from build123d import *

# Parameters (mm, degrees)
SKETCH_1_W          = 104
SKETCH_1_H          = 135
SKETCH_1_R          = 47
EXTRUDE_2_DEPTH     = 100
SKETCH_2_W          = 94
SKETCH_2_H          = 94
CUT_EXTRUDE_1_DEPTH = 95
SKETCH_3_W          = 30
SKETCH_3_H          = 5
SKETCH_3_W_2        = 94
SKETCH_3_H_2        = 20
CUT_EXTRUDE_3_DEPTH = 70
SKETCH_4_W          = 20
SKETCH_4_H          = 4
SKETCH_4_W_2        = 4
SKETCH_4_H_2        = 20
CUT_EXTRUDE_4_DEPTH = 10
CUT_EXTRUDE_6_REACH = 106
SKETCH_6_W          = 55
SKETCH_6_H          = 17
CUT_EXTRUDE_7_REACH = 137
SKETCH_7_W          = 12
SKETCH_7_H          = 12


with BuildPart() as part:
    # 草圖1 → 填料-伸長2 (new body)
    with BuildSketch(Plane.XY):
        with Locations((-20.894077044, -18.213740458)):
            Rectangle(SKETCH_1_W, SKETCH_1_H)
        with Locations((-20.894077044, -7.713740458)):
            Circle(SKETCH_1_R, mode=Mode.SUBTRACT)
    extrude(amount=EXTRUDE_2_DEPTH)

    # 草圖2 → 除料-伸長1 (cut)
    with BuildSketch(Plane.XY.offset(100)):
        with Locations((-20.894077044, -7.713740458)):
            Rectangle(SKETCH_2_W, SKETCH_2_H)
    extrude(amount=-CUT_EXTRUDE_1_DEPTH, mode=Mode.SUBTRACT)

    # 草圖3 → 除料-伸長3 (cut)
    with BuildSketch(Plane.XY.offset(100)):
        with Locations((11.105922956, -57.213740458)):
            Rectangle(SKETCH_3_W, SKETCH_3_H)
        with Locations((-20.894077044, -69.713740458)):
            Rectangle(SKETCH_3_W_2, SKETCH_3_H_2)
    extrude(amount=-CUT_EXTRUDE_3_DEPTH, mode=Mode.SUBTRACT)

    # 草圖4 → 除料-伸長4 (cut)
    with BuildSketch(Plane.XY.offset(100)):
        with Locations((-15.894077044, -81.713740458)):
            Rectangle(SKETCH_4_W, SKETCH_4_H)
        with Locations((28.105922956, -8.713740458)):
            Rectangle(SKETCH_4_W_2, SKETCH_4_H_2)
        with Locations((-15.894077044, 41.286259542)):
            Rectangle(SKETCH_4_W, SKETCH_4_H)
    extrude(amount=-CUT_EXTRUDE_4_DEPTH, mode=Mode.SUBTRACT)

    # 草圖6 → 除料-伸長6 (cut, up to next)
    with BuildSketch(Plane.ZY.offset(72.894077044), mode=Mode.PRIVATE) as cut_extrude_6_sk1:
        with Locations((62.5, 22.786259542)):
            Rectangle(SKETCH_6_W, SKETCH_6_H)
    cut_extrude_6_tool1 = extrude(cut_extrude_6_sk1.sketch, amount=-CUT_EXTRUDE_6_REACH, mode=Mode.PRIVATE) & part.part
    add(cut_extrude_6_tool1.solids().sort_by_distance((-72.894077, 22.78626, 62.5))[0], mode=Mode.SUBTRACT)
    # 草圖6 → 除料-伸長6 (cut, up to next)
    with BuildSketch(Plane.ZY.offset(72.894077044), mode=Mode.PRIVATE) as cut_extrude_6_sk2:
        with Locations((62.5, 1.786259542)):
            Rectangle(SKETCH_6_W, SKETCH_6_H)
    cut_extrude_6_tool2 = extrude(cut_extrude_6_sk2.sketch, amount=-CUT_EXTRUDE_6_REACH, mode=Mode.PRIVATE) & part.part
    add(cut_extrude_6_tool2.solids().sort_by_distance((-72.894077, 1.78626, 62.5))[0], mode=Mode.SUBTRACT)
    # 草圖6 → 除料-伸長6 (cut, up to next)
    with BuildSketch(Plane.ZY.offset(72.894077044), mode=Mode.PRIVATE) as cut_extrude_6_sk3:
        with Locations((62.5, -19.213740458)):
            Rectangle(SKETCH_6_W, SKETCH_6_H)
    cut_extrude_6_tool3 = extrude(cut_extrude_6_sk3.sketch, amount=-CUT_EXTRUDE_6_REACH, mode=Mode.PRIVATE) & part.part
    add(cut_extrude_6_tool3.solids().sort_by_distance((-72.894077, -19.21374, 62.5))[0], mode=Mode.SUBTRACT)
    # 草圖6 → 除料-伸長6 (cut, up to next)
    with BuildSketch(Plane.ZY.offset(72.894077044), mode=Mode.PRIVATE) as cut_extrude_6_sk4:
        with Locations((62.5, -40.213740458)):
            Rectangle(SKETCH_6_W, SKETCH_6_H)
    cut_extrude_6_tool4 = extrude(cut_extrude_6_sk4.sketch, amount=-CUT_EXTRUDE_6_REACH, mode=Mode.PRIVATE) & part.part
    add(cut_extrude_6_tool4.solids().sort_by_distance((-72.894077, -40.21374, 62.5))[0], mode=Mode.SUBTRACT)

    # 草圖7 → 除料-伸長7 (cut, up to next)
    with BuildSketch(Plane.XZ.offset(85.713740458), mode=Mode.PRIVATE) as cut_extrude_7_sk1:
        with Locations((5.105922956, 49)):
            Rectangle(SKETCH_7_W, SKETCH_7_H)
    cut_extrude_7_tool1 = extrude(cut_extrude_7_sk1.sketch, amount=-CUT_EXTRUDE_7_REACH, mode=Mode.PRIVATE) & part.part
    add(cut_extrude_7_tool1.solids().sort_by_distance((5.105923, -85.71374, 49))[0], mode=Mode.SUBTRACT)
    # 草圖7 → 除料-伸長7 (cut, up to next)
    with BuildSketch(Plane.XZ.offset(85.713740458), mode=Mode.PRIVATE) as cut_extrude_7_sk2:
        with Locations((-46.894077044, 49)):
            Rectangle(SKETCH_7_W, SKETCH_7_H)
    cut_extrude_7_tool2 = extrude(cut_extrude_7_sk2.sketch, amount=-CUT_EXTRUDE_7_REACH, mode=Mode.PRIVATE) & part.part
    add(cut_extrude_7_tool2.solids().sort_by_distance((-46.894077, -85.71374, 49))[0], mode=Mode.SUBTRACT)


solid = part.part
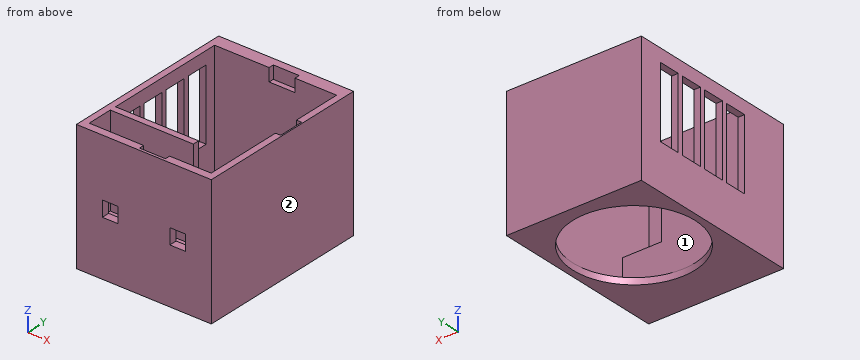
For this review, take the finished solid that the model builds, in its own axes (mm). Face numbers are marked on the shaded views. A direction names the side the tool comes from. Round coordinates to 2 decimals unless told otherwise and drop trailing zeros. Write each loop counter-clockwise with the first axis right and the second up, starting at its lowest first coordinate (ties: lowest second). Pieces come first, ordered by that corner, then holes. Notation, with made-up numbers: M 37.5,-39 L 50.5,-39 A21 cw 50.5,-21 Z; hole C 69.5,29.25 d2. An arc over 180 degrees is marked long. Write item = value, one per line. Start each with the question number.
(1) We need section C-C (x = -48). Give the boundary of the cut face in (y, z).
(2) For line 1 along Y through (x, z) = (-42, 66); line 2 along Y through (x, z) = (24, 22); line 3 along X through (y, z) = (-65, 71), list the stretches that pass through material, from the lowest coordinate up.
(3) We need section B-B (y = -34.5). Give the boundary of the cut face in (x, z), then the cut area to 3 significant figures.
(4) Clearance check with flat-ended pins moving along their axes: pin 1 Ø3 at (y, z) = (18.5, 44.5) entering from -X; pin 2 Ø3 at (x, y) = (-44.5, -81.5) entering from -Z. State where each tip first meets the part, or that it passes through.
(5) We need section D-D (z = 16). Give the boundary of the cut face in (x, y).
(6) For the marked faces 1 and 2, list the 3-axis set-ups (+Z, -Z, +X, -X, +Y, -Y) from which the entire face can be reached by the end or side of a thin tool; tool diameter is ignored.
(7) We need section A-A (z = 59.5). Give the boundary of the cut face in (x, y), then the cut area to 3 significant figures.
Results found:
q1.outline = M -85.71,0 L -46.11,0 L -46.11,5 L -54.71,5 L -54.71,100 L -59.71,100 L -59.71,30 L -79.71,30 L -79.71,43 L -85.71,43 Z; M -85.71,55 L -79.71,55 L -79.71,100 L -85.71,100 Z; M 30.68,0 L 49.29,0 L 49.29,100 L 39.29,100 L 39.29,5 L 30.68,5 Z
q2.line_1 = -85.71 to -79.71, -59.71 to -54.71, 39.29 to 49.29
q2.line_2 = -85.71 to -54.71, 39.29 to 49.29
q2.line_3 = -72.89 to -67.89, 26.11 to 31.11
q3.outline = M -72.89,0 L -59.51,0 L -59.51,5 L -67.89,5 L -67.89,35 L -72.89,35 Z; M -72.89,90 L -67.89,90 L -67.89,100 L -72.89,100 Z; M 17.73,0 L 31.11,0 L 31.11,100 L 26.11,100 L 26.11,5 L 17.73,5 Z
q3.area = 809 mm²
q4.pin_1 = 26.11
q4.pin_2 = 0
q5.outline = M -72.89,-85.71 L 31.11,-85.71 L 31.11,49.29 L -72.89,49.29 Z; hole M -67.89,-54.71 L 26.11,-54.71 L 26.11,39.29 L -67.89,39.29 Z
q6.face_1 = +Z
q6.face_2 = +Z, -Z, +X, +Y, -Y
q7.outline = M -72.89,-85.71 L 31.11,-85.71 L 31.11,49.29 L -72.89,49.29 L -72.89,31.29 L -67.89,31.29 L -67.89,39.29 L 26.11,39.29 L 26.11,-79.71 L -67.89,-79.71 L -67.89,-59.71 L -3.89,-59.71 L -3.89,-54.71 L -67.89,-54.71 L -67.89,-48.71 L -72.89,-48.71 Z; M -72.89,-31.71 L -67.89,-31.71 L -67.89,-27.71 L -72.89,-27.71 Z; M -72.89,-10.71 L -67.89,-10.71 L -67.89,-6.71 L -72.89,-6.71 Z; M -72.89,10.29 L -67.89,10.29 L -67.89,14.29 L -72.89,14.29 Z
q7.area = 2,830 mm²
